Work out the finished part from the listing and answer in its coordinate system (mm). Face numbers are marked on the shaded views. A direction names the side the tool comes from. Coordinates: 2 decimals unless noted, no trailing zeros. Loops run counter-clockwise (first coordinate to the right, second up) from the corner with the lowest first, then second, coordinate; pieces in that order, holes last. Notation, with made-up numbers: (24.25, 69.25) -> (65.25, 69.25) arc R12 ccw to (65.25, 81.25) -> close; hole circle Ø8 at (43, -37.5). An arc over 180 degrees is marked (long way). Use a Markdown table: item, result.
from build123d import *

# Parameters (mm, degrees)
ESBO_O1_W                = 100
ESBO_O1_H                = 120
RESSALTO_EXTRUS_O1_DEPTH = 13
CORTE_EXTRUS_O1_DEPTH    = 12.2
ESBO_O5_W                = 100
ESBO_O5_H                = 120
CORTE_EXTRUS_O2_DEPTH    = 24
CORTE_EXTRUS_O3_DEPTH    = 2.5
ESBO_O7_W                = 1
ESBO_O7_H                = 10
ESBO_O7_W_2              = 1.2
ESBO_O7_W_3              = 10
ESBO_O7_H_2              = 1
ESBO_O7_H_3              = 16.4405419
ESBO_O7_W_4              = 8.5960749
ESBO_O7_H_4              = 1.406812791
RESSALTO_EXTRUS_O2_DEPTH = 1.2
ESBO_O8_W                = 4
ESBO_O8_H                = 4.5
CORTE_EXTRUS_O4_DEPTH    = 10
ESBO_O9_W                = 2
ESBO_O9_H                = 5
RESSALTO_EXTRUS_O3_DEPTH = 2
CHANFRO1_SIZE            = 0.8


with BuildPart() as part:
    # Esboço1 → Ressalto-extrusão1 (new body)
    with BuildSketch(Plane(origin=(0, 0, 0), x_dir=(1, 0, 0), z_dir=(0, 1, 0))):
        with Locations((-3.939393939, -9.393939394)):
            Rectangle(ESBO_O1_W, ESBO_O1_H)
    extrude(amount=RESSALTO_EXTRUS_O1_DEPTH)

    # Esboço2 → Corte-extrusão1 (cut)
    with BuildSketch(Plane(origin=(0, 13, 0), x_dir=(1, 0, 0), z_dir=(0, 1, 0))):
        Polygon((31.508199898, -39.9190402), (31.508199898, 24.595030164), (27.530747921, 28.572482141), (21.431542719, 28.572482141), (19.652327636, 30.351697224), (19.652327636, 33.082043063), (15.960779613, 36.773591087), (7.746138477, 36.773591087), (4.559278928, 39.960450636), (-0.321107452, 39.960450636), (-7.730384523, 32.551173564), (-12.530246006, 32.551173564), (-18.145727819, 26.935691751), (-18.145727819, -12.538643207), (-26.839415482, -3.844955544), (-39.246127252, -3.844955544), (-43.063176727, -7.662005018), (-43.063176727, -20.068716788), (-7.730384523, -55.401508991), (15.960779613, -55.401508991), align=None)
    extrude(amount=-CORTE_EXTRUS_O1_DEPTH, mode=Mode.SUBTRACT)

    # Esboço5 → Corte-extrusão2 (cut)
    with BuildSketch(Plane(origin=(0, 13, 0), x_dir=(1, 0, 0), z_dir=(0, 1, 0))):
        with Locations((-3.939393939, -9.393939394)):
            Rectangle(ESBO_O5_W, ESBO_O5_H)
        Polygon((34.008199898, 16.264683084), (34.008199898, 25.63056407), (28.566281827, 31.072482141), (22.467076625, 31.072482141), (22.152327636, 31.38723113), (22.152327636, 34.117576969), (16.996313518, 39.273591087), (8.781672383, 39.273591087), (5.594812834, 42.460450636), (-1.356641358, 42.460450636), (-8.765918429, 35.051173564), (-13.565779912, 35.051173564), (-20.645727819, 27.971225657), (-20.645727819, -6.503109301), (-25.803881576, -1.344955544), (-40.281661158, -1.344955544), (-45.563176727, -6.626471112), (-45.563176727, -21.104250694), (-8.765918429, -57.901508991), (9.20558363, -57.901508991), (16.993249442, -57.901508991), (34.008199898, -40.95764084), align=None, mode=Mode.SUBTRACT)
    extrude(amount=-CORTE_EXTRUS_O2_DEPTH, mode=Mode.SUBTRACT)

    # Esboço6 → Corte-extrusão3 (cut)
    with BuildSketch(Plane(origin=(0, 13, 0), x_dir=(1, 0, 0), z_dir=(0, 1, 0))):
        Polygon((-26.42520192, -2.844955544), (-19.145727819, -10.124429645), (-19.145727819, 27.349905314), (-12.944459568, 33.551173564), (-8.144598086, 33.551173564), (-0.735321014, 40.960450636), (4.97349249, 40.960450636), (8.160352039, 37.773591087), (16.374993175, 37.773591087), (20.652327636, 33.496256625), (20.652327636, 30.765910786), (21.845756281, 29.572482141), (27.944961483, 29.572482141), (32.508199898, 25.009243726), (32.508199898, -40.708099195), (16.814790102, -56.401508991), (-8.144598086, -56.401508991), (-44.063176727, -20.48293035), (-44.063176727, -7.247791456), (-39.660340814, -2.844955544), align=None)
    extrude(amount=-CORTE_EXTRUS_O3_DEPTH, mode=Mode.SUBTRACT)

    # Esboço7 → Ressalto-extrusão2 (add)
    with BuildSketch(Plane(origin=(0, 13, 0), x_dir=(1, 0, 0), z_dir=(0, 1, 0))):
        with Locations((-18.645727819, 5)):
            Rectangle(ESBO_O7_W, ESBO_O7_H)
        with Locations((31.908199898, -33.775847323)):
            Rectangle(ESBO_O7_W_2, ESBO_O7_H)
        with Locations((31.908199898, 18.926155897)):
            Rectangle(ESBO_O7_W_2, ESBO_O7_H)
        with Locations((7.086788937, -55.901508991)):
            Rectangle(ESBO_O7_W_3, ESBO_O7_H_2)
        with Locations((-43.469924349, -13.990706428)):
            Rectangle(ESBO_O7_W_2, ESBO_O7_H_3)
        Polygon((-27.607092583, -36.939014494), (-20.536024771, -44.010082306), (-19.687496633, -43.161554169), (-26.758564445, -36.090486357), align=None)
        with Locations((2.082267831, 40.257044241)):
            Rectangle(ESBO_O7_W_4, ESBO_O7_H_4)
    extrude(amount=-RESSALTO_EXTRUS_O2_DEPTH)

    # Esboço8 → Corte-extrusão4 (cut)
    with BuildSketch(Plane.XY.offset(57.901508991)):
        with Locations((-10.765918429, 10.75)):
            Rectangle(ESBO_O8_W, ESBO_O8_H)
    extrude(amount=-CORTE_EXTRUS_O4_DEPTH, mode=Mode.SUBTRACT)

    # Esboço9 → Ressalto-extrusão3 (add)
    with BuildSketch(Plane(origin=(0, 0.8, 0), x_dir=(1, 0, 0), z_dir=(0, 1, 0))):
        with Locations((1.570718191, 31.875055196)):
            Rectangle(ESBO_O9_W, ESBO_O9_H)
    extrude(amount=RESSALTO_EXTRUS_O3_DEPTH)

    # Chanfro1
    chanfro1_edges = [part.edges().sort_by_distance(p)[0] for p in [
        (-18.145727819, 13, -5),
        (7.086788937, 13, 55.401508991),
        (31.308199898, 13, 33.775847323),
        (-23.223030539, 13, 39.626020263),
        (2.119085738, 13, -39.553637845),
        (31.308199898, 13, -18.926155897),
    ]]
    chamfer(chanfro1_edges, length=CHANFRO1_SIZE)


solid = part.part
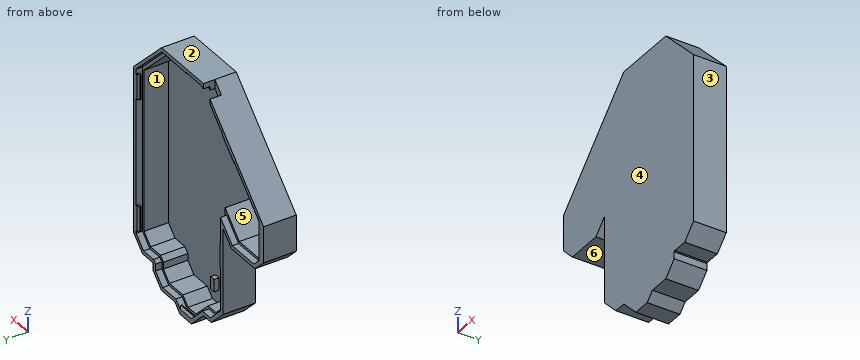
Q1. For the marked faces 4, 5 and 6, determine the directions among +Z, -Z, +X, -X, +Y, -Y from which every point of the face is accessible in a straight line to the end or side of a thin tool.
Solved:
| item | result |
|---|---|
| face 4 | +Z, -Z, +X, -X, -Y |
| face 5 | +Y |
| face 6 | -Z, -X, +Y, -Y |
Q2. Given pin 1 Ø4 at (y, z) = (3.5, -13.5) entering from -X; pin 2 Ø0.8 at (x, y) = (-10, 12) entering from +Z; pin 3 Ø4 at (x, z) = (6, -2.5) entering from +Y, each flat-ended and moving along its own axis, determine where each tip first touches the part or whether it passes through.
Solved:
| item | result |
|---|---|
| pin 1 | x = -20.65 |
| pin 2 | z = -33.55 |
| pin 3 | y = 0.8 |
Q3. Section C-C on z = 33 is taken. Determine the outline of the cut face in (x, y), and give its area (3 significant figures).
Solved:
| item | result |
|---|---|
| outline | (-33.67, 0) -> (34.01, 0) -> (34.01, 13) -> (32.11, 13) -> (31.31, 12.2) -> (31.31, 11.8) -> (32.51, 11.8) -> (32.51, 10.5) -> (31.51, 10.5) -> (31.51, 0.8) -> (-30.13, 0.8) -> (-30.13, 10.5) -> (-31.55, 10.5) -> (-31.55, 13) -> (-33.67, 13) -> close |
| area | 123 mm² |
Q4. Consider line 1 (X direction, y = 9.25, z = 11); line 2 (X direction, y = 8.5, z = 2); line 3 (Z direction, x = 14.5, y = 7.25). Determine where each line is inside the solid, lowest interval first. Write a range as [from, to].
Solved:
| item | result |
|---|---|
| line 1 | [-45.56, -43.06], [-19.68, -18.15], [31.51, 34.01] |
| line 2 | [-40.94, -25.15], [-20.65, -18.15], [31.51, 34.01] |
| line 3 | [-39.27, -36.77], [55.4, 57.9] |
Q5. Section B-B on z = -21 is taken. Determine the outline of the cut face in (x, y).
Solved:
| item | result |
|---|---|
| outline | (-20.65, 0) -> (34.01, 0) -> (34.01, 13) -> (32.11, 13) -> (31.31, 12.2) -> (31.31, 11.8) -> (32.51, 11.8) -> (32.51, 10.5) -> (31.51, 10.5) -> (31.51, 0.8) -> (-18.15, 0.8) -> (-18.15, 10.5) -> (-19.15, 10.5) -> (-19.15, 13) -> (-20.65, 13) -> close |
Q6. Determine the mould class of the marked faces 1, 2 and 3 for opening direction Z: pulls with the +Z half, pulls with the -Z half, needs draft (parallel to the pull), parting line crosses it, or undercut.
Solved:
| item | result |
|---|---|
| face 1 | undercut |
| face 2 | pulls with the +Z half |
| face 3 | needs draft |
Q7. Section D-D on x = -35 is taken. Determine the outline of the cut face in (y, z).
Solved:
| item | result |
|---|---|
| outline | (0, 1.34) -> (13, 1.34) -> (13, 2.84) -> (10.5, 2.84) -> (10.5, 3.84) -> (0.8, 3.84) -> (0.8, 28.13) -> (10.5, 28.13) -> (10.5, 29.55) -> (13, 29.55) -> (13, 31.67) -> (0, 31.67) -> close |
Q8. Section A-A on x = 18.5 is taken. Determine the outline of the cut face in (y, z).
Solved:
| item | result |
|---|---|
| outline | (0, -37.77) -> (13, -37.77) -> (13, -35.65) -> (10.5, -35.65) -> (10.5, -34.23) -> (0.8, -34.23) -> (0.8, 52.87) -> (10.5, 52.87) -> (10.5, 54.72) -> (13, 54.72) -> (13, 56.4) -> (0, 56.4) -> close |
